Check sheet for the modelled part. Datum: model origin and axes. Units: mm. A direction names the side the tool comes from. Give positions to 0.01 mm unless a question says otherwise; leave off trailing zeros. Write each loop counter-clockwise with the first axis right and the second up, starting at its lowest first coordinate (ties: lowest second). Pieces come first, ordered by that corner, then holes. Notation, with made-up numbers: (53.25, 59.5) -> (104.25, 59.5) arc R22 cw to (104.25, 94.5) -> close; hole circle Ø2 at (-25.5, 75.5). An arc over 180 degrees is marked (long way). Return JSON: item names as keys, results as strings.
from build123d import *

# Parameters (mm, degrees)
F1_DEPTH = 63.5
F2_T     = -2.54
F3_R     = 6.35
F4_DEPTH = 95.25


with BuildPart() as f1:
    # F0 (on Top) → F1 (new body)
    with BuildSketch(Plane.XY):
        Polygon((97.79, 104.14), (0, 104.14), (-97.79, 104.14), (-97.79, -104.14), (97.79, -104.14), (97.79, 0), align=None)
    extrude(amount=F1_DEPTH)

    # F2
    f2_openings = [f1.faces().sort_by_distance(p)[0] for p in [
        (0, 0, 63.5),
    ]]
    offset(amount=F2_T, openings=f2_openings)

    # F3 (on face) → F4 (join)
    with BuildSketch(Plane.XY.offset(2.54)):
        with Locations((23.5758665949, 35.8260651119)):
            Circle(F3_R)
        with Locations((-23.5758665949, -35.8260651119)):
            Circle(F3_R)
    extrude(amount=F4_DEPTH)


solid = f1.part
(1) Depth check by flat-ended pin: pin 1 Ø3 at (x, z) = (28.5, 77.5) entering from +Y; pin 2 Ø10 at (y, z) = (-55, 71.5) entering from +X; pin 3 Ø6 at (x, y) = (-70, 69.5) entering from +Z; pin 4 Ø1.5 at (x, y) = (64, 32.5) entering from -Z. Enter the tip coordinate at first touch or a pass-through.
Reply:
{"pin 1": "y = 41.17", "pin 2": "through", "pin 3": "z = 2.54", "pin 4": "z = 0"}
(2) Cross-section at B-B on x = 50.5. Enter the section's corners in (y, z).
Reply:
{"outline": "(-104.14, 0) -> (104.14, 0) -> (104.14, 63.5) -> (101.6, 63.5) -> (101.6, 2.54) -> (-101.6, 2.54) -> (-101.6, 63.5) -> (-104.14, 63.5) -> close"}
(3) Set-up check for faces 5 (the flat face through (23, 36, 97.79)), 6 (the cylindrical face through (-17.52, -33.92, 49.5)): record each of +Z, -Z, +X, -X, +Y, -Y from which the full face is reachable in a straight line by a thin tool's end or side.
Reply:
{"face 5": "+Z, +X, -X, +Y, -Y", "face 6": "+Z"}
(4) Cross-section at D-D on z = 70.5. Enter the section's corners in (x, y).
Reply:
{"outline": "circle Ø12.7 at (-23.58, -35.83); circle Ø12.7 at (23.58, 35.83)"}
(5) Release check for a two-part mould opening along X. For faces 1 (the flat face through (-97.79, 1, 31)), 2 (the flat face through (-1, -104.14, 31)), 3 (the flat face through (-1, -101.6, 33)), 4 (the flat face through (-1, 1, 2.54)) record: pulls with the +X half, pulls with the -X half, needs draft (parallel to the pull), parting line crosses it, or undercut.
Reply:
{"face 1": "pulls with the -X half", "face 2": "needs draft", "face 3": "undercut", "face 4": "undercut"}
(6) Thickness scan on L1, parallel to X at y = 57, z = 50; L2, parallel to Y at x = 77, z = 59; L3, parallel to Z at x = 50.5, y = 22.5. Record the ranges inside material, lowest first.
Reply:
{"L1": "-97.79 to -95.25, 95.25 to 97.79", "L2": "-104.14 to -101.6, 101.6 to 104.14", "L3": "0 to 2.54"}
(7) Cross-section at C-C on y = -83.5. Enter the section's corners in (x, z).
Reply:
{"outline": "(-97.79, 0) -> (97.79, 0) -> (97.79, 63.5) -> (95.25, 63.5) -> (95.25, 2.54) -> (-95.25, 2.54) -> (-95.25, 63.5) -> (-97.79, 63.5) -> close"}
(8) Cross-section at A-A on z = 54. Enter the section's corners in (x, y), then the cut area to 3 significant figures.
Reply:
{"outline": "(-97.79, -104.14) -> (97.79, -104.14) -> (97.79, 104.14) -> (-97.79, 104.14) -> close; circle Ø12.7 at (-23.58, -35.83); circle Ø12.7 at (23.58, 35.83); hole (-95.25, -101.6) -> (95.25, -101.6) -> (95.25, 101.6) -> (-95.25, 101.6) -> close", "area": "2,280 mm^2"}
